Read the model definition and answer for the solid it produces. Units are mm, in the model's axes. A direction names the side the tool comes from. Round coordinates to 2 decimals unless told otherwise and drop trailing zeros. Loops run counter-clockwise (first coordinate to the right, second up) from the corner with the lowest first, then second, coordinate; pieces in that order, holes last. Notation, with made-up numbers: (-38.75, -33.5) - (8.25, -33.5) arc R18 cw to (8.25, -13.5) - close; hole circle Ø11 at (82, 65.5). An arc over 180 degrees is marked (long way). Use CSV: the item, a comma, the result in double quotes. Start each with the question number.
1. Given pin 1 Ø4 at (y, z) = (17.96, -17.96) entering from -X; pin 2 Ø2 at (x, z) = (1.5, -22.5) entering from +Y, each flat-ended and moving along its own axis, determine where each tip first touches the part or whether it passes through.
2. Determine the mould class of faces 3 (the cylindrical face through (3.22, -0.54, -27.83)), 4 (the flat face through (3, -109, 50.8)), 5 (the flat face through (3, -227.006, 26)) for opening direction Y: +Y half, -Y half, draft (parallel to the pull), parting line (faces both ways), or undercut.
3. Find section C-C (x = 3). State how many separate pieces and enclosed holes the cut face has, and give its area (3 significant figures).
4. Find section D-D (z = 25.4). Give the vertices of the cut face in (x, y), and give its area (3 significant figures).
5. Find section A-A (y = -146.05). Give the vertices of the cut face in (x, z).
6. Consider line 1 along Y through (x, z) = (4, 5.5); line 2 along Y through (x, z) = (2.5, 24) (1 decimal); line 3 along Z through (x, y) = (3.5, -146.05). Determine where each line is inside the solid, lowest interval first.
7. A tool of negligible diameter and unlimited length cuts with its end or side. For faces 1 (the flat face through (3, -216, 0)), 2 (the flat face through (3, -96, -50.8)), from which of +Z, -Z, +X, -X, +Y, -Y can it reach the whole face along a straight path? Write none if from no direction.
8. Find section B-B (z = -25.4). Give the vertices of the cut face in (x, y).
from build123d import *
from build123d.topology import SkipClean

# Parameters (mm, degrees)
SKETCH1_R                  = 14.2875
BOSS_EXTRUDE1_DEPTH        = 6.35
F_0_257_DIAMETER_HOLE1_D   = 6.5278
F_9_0_196_DIAMETER_HOLE1_D = 4.9784
F_9_0_196_DIAMETER_HOLE2_D = 4.9784
BOSS_EXTRUDE3_START        = -6.35
BOSS_EXTRUDE3_DEPTH        = 6.35
CUT_EXTRUDE1_START         = -6.35
SKETCH11_R                 = 14.2875
CUT_EXTRUDE1_DEPTH         = 6.35
FILLET1_R                  = 6.35


with BuildPart() as part:
    # Sketch1 → Boss-Extrude1 (new body)
    with BuildSketch(Plane.YZ):
        with BuildLine():
            Line((0, -50.8), (-198.714420778, -50.8))
            ThreePointArc((-198.714420778, -50.8), (-205.105, 0), (-198.714420778, 50.8))
            Line((-198.714420778, 50.8), (0, 50.8))
            ThreePointArc((0, 50.8), (50.8, 0), (0, -50.8))
        make_face()
        with Locations(Location((0, 0, 0), (0, 0, 270))):
            Circle(SKETCH1_R, mode=Mode.SUBTRACT)
        with Locations(Location((-33.782, 0, 0), (0, 0, 270))):
            Circle(SKETCH1_R, mode=Mode.SUBTRACT)
    extrude(amount=BOSS_EXTRUDE1_DEPTH)

    # F (0.257) Diameter Hole1 (through all)
    with Locations(Plane.YZ.offset(6.35)):
        with Locations((0, 0), (-190.721063402, -25.4), (-192.209068041, -8.680909393), (-187.906487547, 41.362252872)):
            Hole(F_0_257_DIAMETER_HOLE1_D / 2)

    # #9 (0.196) Diameter Hole1 (through all)
    with Locations(Plane.YZ.offset(6.35)):
        with Locations((-146.05, 38.1), (-69.85, 38.1)):
            Hole(F_9_0_196_DIAMETER_HOLE1_D / 2)

    # #9 (0.196) Diameter Hole2 (through all)
    with Locations(Plane(origin=(0, 0, 0), x_dir=(0, -1, 0), z_dir=(-1, 0, 0))):
        with Locations((59.182, 0), (0, 25.4), (0, -25.4), (-17.960512242, -17.960512242), (-17.960512242, 17.960512242)):
            Hole(F_9_0_196_DIAMETER_HOLE2_D / 2)

    # Sketch10 → Boss-Extrude3 (add)
    with BuildSketch(Plane.YZ.offset(6.35).offset(BOSS_EXTRUDE3_START)):
        with BuildLine():
            Line((-198.714420778, 50.8), (-227.006249903, 50.8))
            Line((-227.006249903, 50.8), (-227.006249903, 0))
            Line((-227.006249903, 0), (-205.105, 0))
            ThreePointArc((-205.105, 0), (-205.024737282, 5.737432126), (-204.784011946, 11.470373851))
            ThreePointArc((-204.784011946, 11.470373851), (-215.781689349, 27.1859375), (-201.229613759, 39.68253484))
            Line((-201.229613759, 39.68253484), (-198.714420778, 50.8))
        make_face()
    extrude(amount=BOSS_EXTRUDE3_DEPTH)

    # Sketch11 → Cut-Extrude1 (cut)
    with SkipClean():  # the faces are left unmerged after this step: merging them gives an invalid solid
        with BuildSketch(Plane.YZ.offset(6.35).offset(CUT_EXTRUDE1_START)):
            with Locations(Location((-201.606249903, 25.4, 0), (0, 0, 90))):
                Circle(SKETCH11_R)
        extrude(amount=CUT_EXTRUDE1_DEPTH, mode=Mode.SUBTRACT)

    # Fillet1
    fillet1_edges = [part.edges().sort_by_distance(p)[0] for p in [
        (3.175, -198.714420778, -50.8),
        (3.175, -205.105, 0),
        (3.175, -227.006249903, 0),
        (3.175, -227.006249903, 50.8),
    ]]
    fillet(fillet1_edges, radius=FILLET1_R)


solid = part.part
Filled sheet:
1,pin 1,"passes through"
1,pin 2,"stops at y = 46.03"
2,face 3,"undercut"
2,face 4,"draft"
2,face 5,"-Y half"
3,separate pieces,"1"
3,enclosed holes,"13"
3,area,"23,700 mm²"
4,outline,"(0, -227.01) - (6.35, -227.01) - (6.35, -215.89) - (0, -215.89) - close; (0, -187.32) - (6.35, -187.32) - (6.35, -2.49) - (0, -2.49) - close; (0, 2.49) - (6.35, 2.49) - (6.35, 43.99) - (0, 43.99) - close"
4,area,"1,510 mm²"
5,outline,"(0, -50.8) - (6.35, -50.8) - (6.35, 35.61) - (0, 35.61) - close; (0, 40.59) - (6.35, 40.59) - (6.35, 50.8) - (0, 50.8) - close"
6,line 1,"y = -226.95 to -46.97, -20.6 to -13.19, 13.19 to 50.5"
6,line 2,"y = -227 to -215.8, -187.4 to -2.1, 2.1 to 44.8"
6,line 3,"z = -50.8 to 35.61, 40.59 to 50.8"
7,face 1,"-Z, +X, -X, -Y"
7,face 2,"-Z, +X, -X, +Y, -Y"
8,outline,"(0, -203.53) - (6.35, -203.53) - (6.35, -193.98) - (0, -193.98) - close; (0, -187.46) - (6.35, -187.46) - (6.35, -2.49) - (0, -2.49) - close; (0, 2.49) - (6.35, 2.49) - (6.35, 43.99) - (0, 43.99) - close"
